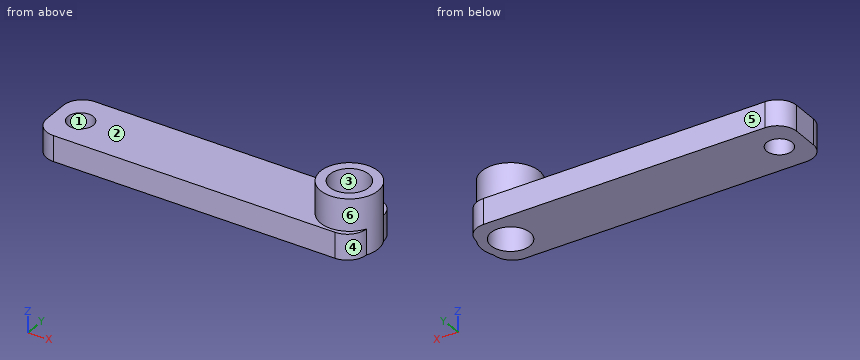
from build123d import *

# Parameters (mm, degrees)
SKETCH_1_W           = 50
SKETCH_1_H           = 10
SKETCH_1_R           = 3.05
SKETCH_1_R_2         = 2
EXTRUDE_1_DEPTH      = 4
EXTRUDE_2_DEPTH      = 5
EXTRUDE_2_DEPTH_BACK = 4
SKETCH_2_R           = 4.5
SKETCH_2_R_2         = 3.05
FILLET_1_R           = 3


with BuildPart() as part:
    # 草图1 → 凸台-拉伸1 (new body)
    with BuildSketch(Plane.XY):
        Rectangle(SKETCH_1_W, SKETCH_1_H)
        with Locations((21, 0)):
            Circle(SKETCH_1_R, mode=Mode.SUBTRACT)
        with Locations((-21, 0)):
            Circle(SKETCH_1_R_2, mode=Mode.SUBTRACT)
    extrude(amount=EXTRUDE_1_DEPTH)

    # 草图2 → 凸台-拉伸2 (add, two sides: drawn at the far end of the back side and taken through both)
    with BuildSketch(Plane.XY.offset(4).offset(-EXTRUDE_2_DEPTH_BACK)):
        with Locations((21, 0)):
            Circle(SKETCH_2_R)
        with Locations((21, 0)):
            Circle(SKETCH_2_R_2, mode=Mode.SUBTRACT)
    extrude(amount=EXTRUDE_2_DEPTH + EXTRUDE_2_DEPTH_BACK)

    # 圆角1
    # the kernel refuses this fillet: 3 mm, written as the material it takes off along each edge
    with BuildSketch(Plane(origin=(25, -5, -7.5), x_dir=(-1, 0, 0), z_dir=(0, 0, 1))) as fillet_1_piece_1_section:
        with BuildLine():
            CenterArc((FILLET_1_R, -FILLET_1_R), FILLET_1_R, 90, 90)
            Line((0, -FILLET_1_R), (0, 0))
            Line((0, 0), (FILLET_1_R, 0))
        make_face()
    fillet_1_piece_1 = extrude(amount=19, mode=Mode.PRIVATE)
    fillet_1_piece_1 = fillet_1_piece_1 - Plane(origin=(21, 0, 2), x_dir=(1, 0, 0), z_dir=(0, 0, 1)) * Cylinder(4.5, 50, mode=Mode.PRIVATE)
    add(fillet_1_piece_1, mode=Mode.SUBTRACT)
    with BuildSketch(Plane(origin=(25, 5, -7.5), x_dir=(-1, 0, 0), z_dir=(0, 0, 1))) as fillet_1_piece_2_section:
        with BuildLine():
            CenterArc((FILLET_1_R, FILLET_1_R), FILLET_1_R, 180, 90)
            Line((0, FILLET_1_R), (0, 0))
            Line((0, 0), (FILLET_1_R, 0))
        make_face()
    fillet_1_piece_2 = extrude(amount=19, mode=Mode.PRIVATE)
    fillet_1_piece_2 = fillet_1_piece_2 - Plane(origin=(21, 0, 2), x_dir=(1, 0, 0), z_dir=(0, 0, 1)) * Cylinder(4.5, 50, mode=Mode.PRIVATE)
    add(fillet_1_piece_2, mode=Mode.SUBTRACT)
    with BuildSketch(Plane(origin=(-25, -5, -7.5), x_dir=(0, 1, 0), z_dir=(0, 0, 1)), Plane(origin=(-25, 5, -7.5), x_dir=(1, 0, 0), z_dir=(0, 0, 1))) as fillet_1_piece_3:
        with BuildLine():
            CenterArc((FILLET_1_R, -FILLET_1_R), FILLET_1_R, 90, 90)
            Line((0, -FILLET_1_R), (0, 0))
            Line((0, 0), (FILLET_1_R, 0))
        make_face()
    extrude(amount=19, mode=Mode.SUBTRACT)


solid = part.part
Can you work these out from the model? Positions are in its coordinate system, mm. Face numbers are marked on the shaded views. A direction names the side the tool comes from. Round coordinates to 2 decimals unless told otherwise and drop trailing zeros. Write each loop counter-clockwise with the first axis right and the second up, starting at its lowest first coordinate (ties: lowest second). Pieces come first, ordered by that corner, then holes. Notation, with made-up numbers: (19.25, -15) -> (48.25, -15) arc R22 cw to (48.25, 0) -> close; hole circle Ø6 at (-25, 38.5). An arc over 180 degrees is marked (long way). Use one line per item in the form item = value. Start each with the question number.
Q1. If I drill on probe 1 along Y at (x, z) = (-21, 1.7); probe 2 along Y at (x, z) = (21, 2.25); probe 3 along Z at (x, y) = (9, 1.25), over which ranges is the centre line in solid material (lowest first)? Write a range as [from, to].
Q2. Which directions (+Z, -Z, +X, -X, +Y, -Y) give clear straight access to the entire face, cutting with the end or side of a thin tool? Please do the marked faces 5 and 6.
Q3. I'm going to push flat-ended pins straight in: P1, Ø3.5, axis at x = -21, y = 0, coming from the +Z side; P2, Ø4, axis at y = 0.5, z = 8, coming from the +X side; P3, Ø3, axis at y = 3, z = 7.5, coming from the +X side. Where does each tip first touch, or does it pass through?
Q4. Imagine slicing it at D-D (x = -21). Please give me the cut outline in (y, z), then the cut area to 3 significant figures.
Q5. Imagine slicing it at C-C (z = 2.25). Please give me the cut outline in (x, y).
Q6. Imagine slicing it at A-A (x = 21). Please give me the cut outline in (y, z).
Q7. We'd pull the mould along X, two halves only. Please class the marked faces 1, 2, 3 and 4: +X half, -X half, draft (parallel to the pull), parting line (faces both ways), or undercut.
Q8. Imagine slicing it at B-B (y = 0). Please give me the cut outline in (x, z).
Worked out:
q1.probe_1 = [-5, -2], [2, 5]
q1.probe_2 = [-5, -3.05], [3.05, 5]
q1.probe_3 = [0, 4]
q2.face_5 = +Z, -Z, +X, -X, +Y
q2.face_6 = +Z
q3.P1 = through
q3.P2 = 25.5
q3.P3 = 25.24
q4.outline = (-5, 0) -> (-2, 0) -> (-2, 4) -> (-5, 4) -> close; (2, 0) -> (5, 0) -> (5, 4) -> (2, 4) -> close
q4.area = 24.0 mm^2
q5.outline = (-25, -2) arc R3 ccw to (-22, -5) -> (22, -5) arc R3 ccw to (25, -2.06) arc R4.5 ccw to (25, 2.06) arc R3 ccw to (22, 5) -> (-22, 5) arc R3 ccw to (-25, 2) -> close; hole circle Ø4 at (-21, 0); hole circle Ø6.1 at (21, 0)
q6.outline = (-5, 0) -> (-3.05, 0) -> (-3.05, 9) -> (-4.5, 9) -> (-4.5, 4) -> (-5, 4) -> close; (3.05, 0) -> (5, 0) -> (5, 4) -> (4.5, 4) -> (4.5, 9) -> (3.05, 9) -> close
q7.face_1 = undercut
q7.face_2 = draft
q7.face_3 = undercut
q7.face_4 = +X half
q8.outline = (-25, 0) -> (-23, 0) -> (-23, 4) -> (-25, 4) -> close; (-19, 0) -> (17.95, 0) -> (17.95, 9) -> (16.5, 9) -> (16.5, 4) -> (-19, 4) -> close; (24.05, 0) -> (25.5, 0) -> (25.5, 9) -> (24.05, 9) -> close
